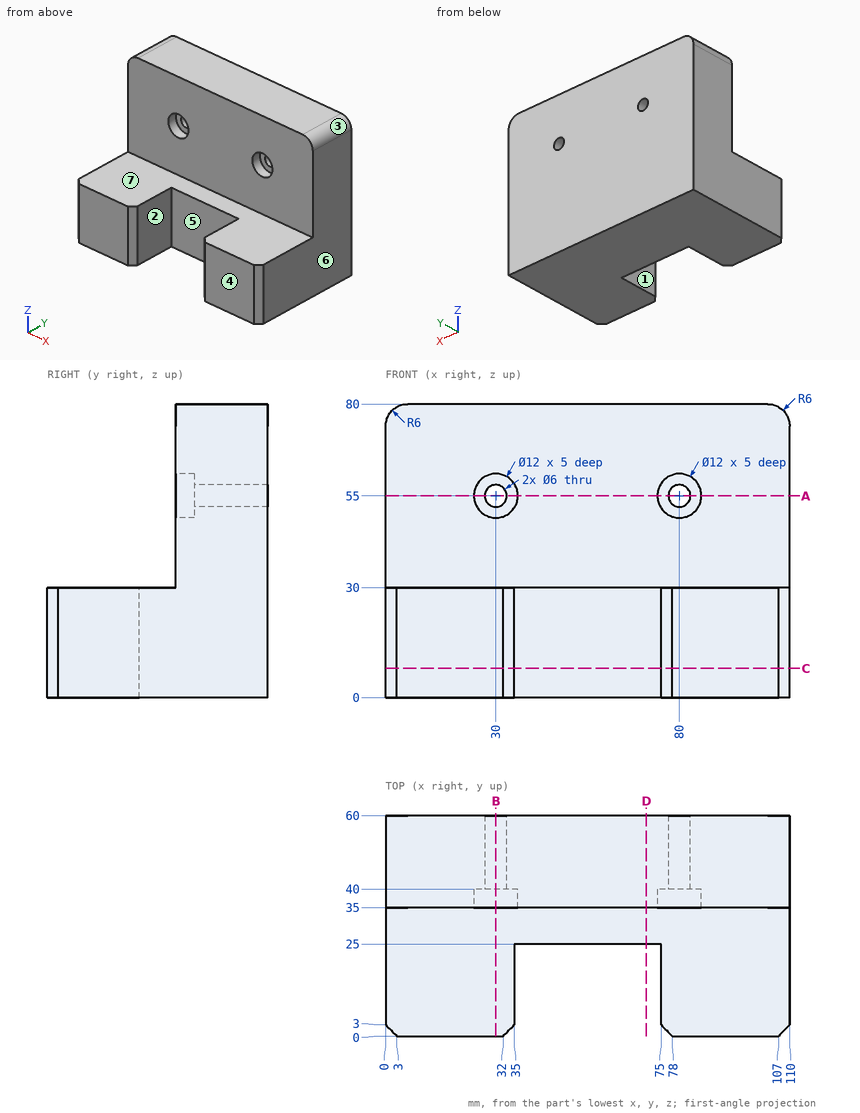
Here's the drawing with two shaded views (mm, measured from the low corner). I have some questions. A direction names the side the tool comes from. Coordinates: 2 decimals unless noted, no trailing zeros. Order: outer loops, then holes, each group sorted by start corner. A loop starts at its lowest first (then second) coordinate and runs counter-clockwise, first axis right, second up.
Q1. Suppose I cut it at C-C on z = 8. Please give me the cut outline in (x, y), and give its area (3 significant figures).
Q2. Thinking about a two-plate mould opening in X: for the marked faces 1, 2, 3 and 4, which applies, released by +X, released by -X, zero draft, split by the parting line, or undercut?
Q3. Suppose I cut it at D-D on x = 71. Please give me the cut outline in (y, z), and give its area (3 significant figures).
Q4. Suppose I cut it at B-B on x = 30. Please give me the cut outline in (y, z).
Q5. Please list where these lines run through material, in increasing order: L1, parallel to Z at x = 30, y = 36.7; L2, parallel to X at y = 35.5, z = 52; L3, parallel to X at y = 3, z = 24.5.
Q6. Will these pins go through, and if not, where does the flat tip stop? pin 1 (17.5 mm diameter, centred on x = 33, y = 17.5, fed in from +Z); pin 2 (25 mm diameter, centred on x = 43, z = 53, fed in from -Y); pin 3 (5 mm diameter, centred on x = 80, z = 55, fed in from +Y); pin 4 (1 mm diameter, centred on x = 94, y = 46, fed in from -Z).
Q7. Which directions (+Z, -Z, +X, -X, +Y, -Y) give clear straight access to the entire face, cutting with the end or side of a thin tool? Please do the marked faces 5, 6 and 7.
Q8. Suppose I cut it at A-A on z = 55. Please give me the cut outline in (x, y).
Answer:
1. outline: (0, 3) - (3, 0) - (32, 0) - (35, 3) - (35, 25) - (75, 25) - (75, 3) - (78, 0) - (107, 0) - (110, 3) - (110, 60) - (0, 60) - close
1. area: 5,580 mm2
2. face 1: undercut
2. face 2: undercut
2. face 3: released by +X
2. face 4: zero draft
3. outline: (25, 0) - (60, 0) - (60, 80) - (35, 80) - (35, 30) - (25, 30) - close
3. area: 2,300 mm2
4. outline: (0, 0) - (60, 0) - (60, 52) - (40, 52) - (40, 49) - (35, 49) - (35, 30) - (0, 30) - close; (35, 61) - (40, 61) - (40, 58) - (60, 58) - (60, 80) - (35, 80) - close
5. L1: z = 0 to 49, 61 to 80
5. L2: x = 0 to 24.8, 35.2 to 74.8, 85.2 to 110
5. L3: x = 0 to 35, 75 to 110
6. pin 1: stops at z = 30
6. pin 2: stops at y = 35
6. pin 3: passes through
6. pin 4: stops at z = 0
7. face 5: +Z, -Z, -Y
7. face 6: +Z, -Z, +X, +Y, -Y
7. face 7: +Z, +X, -X, -Y
8. outline: (0, 35) - (24, 35) - (24, 40) - (27, 40) - (27, 60) - (0, 60) - close; (33, 40) - (36, 40) - (36, 35) - (74, 35) - (74, 40) - (77, 40) - (77, 60) - (33, 60) - close; (83, 40) - (86, 40) - (86, 35) - (110, 35) - (110, 60) - (83, 60) - close
